Can you work these out from the model? Positions are in its coordinate system, mm. A direction names the side the tool comes from. Round coordinates to 2 decimals unless told otherwise and drop trailing zeros. Write each loop counter-clockwise with the first axis right and the second up, starting at its lowest first coordinate (ties: lowest second). Pieces come first, ordered by that corner, then holes. Notation, with made-up numbers: M 68,-22 L 123,-22 A14 ccw 123,-9 Z; hole C 52,48 d8. An arc over 180 degrees is marked long. Answer as a JSON object with one key per item and string values. Group by question number.
1) I'm going to push flat-ended pins straight in: pin 1 Ø6 at (x, z) = (-2, 7.5) entering from +Y; pin 2 Ø1 at (x, z) = (-2, 8.5) entering from -Y; pin 3 Ø5.5 at (x, y) = (-2, 4.5) entering from +Z; pin 4 Ø2 at (x, z) = (-6.5, 9.5) entering from -Y. Where does each tip first touch, or does it pass through?
2) Suppose I cut it at B-B, the plane y = -7.75. Write out the boundary of the cut face in (x, z).
3) Suppose I cut it at D-D, the plane z = 7. Write out the boundary of the cut face in (x, y), and give its area (3 significant figures).
4) Please list where these lines run through material, in increasing order: L1, parallel to Z at x = -6, y = -3.5; L2, parallel to X at y = -0.25, z = 21.5; L3, parallel to X at y = -5, z = 2 (3 decimals). Write a range as [from, to].
5) Suppose I cut it at C-C, the plane x = -6.25. Write out the boundary of the cut face in (y, z).
6) Suppose I cut it at A-A, the plane z = 2.5. Write out the boundary of the cut face in (x, y), and give its area (3 significant figures).
7) On a 3-axis mill with a long thin cutter (end or side, diameter ignored), from which of +Z, -Z, +X, -X, +Y, -Y can I reach the whole of each face in a straight line? I mean faces 1 (the flat face through (-8.665, -0.488, 1.972)), 2 (the cylindrical face through (-0.867, -3.905, 13.381)). Say none if no direction works.
from build123d import *

# Parameters (mm, degrees)
EXTRUDE_3_DEPTH = 4
SKETCH_3_R      = 4
EXTRUDE_4_DEPTH = 20
FILLET_1_R      = 1
FILLET_2_R      = 2


with BuildPart() as part:
    # 草图1 → 凸台-拉伸3 (new body)
    with BuildSketch(Plane.XY):
        Polygon((-8.337851922, -5.558416845), (0.644804231, -10), (8.982656153, -4.441583155), (8.337851922, 5.558416845), (-0.644804231, 10), (-8.982656153, 4.441583155), align=None)
    extrude(amount=EXTRUDE_3_DEPTH)

    # 草图3 → 凸台-拉伸4 (add)
    with BuildSketch(Plane.XY.offset(4)):
        Circle(SKETCH_3_R)
    extrude(amount=EXTRUDE_4_DEPTH)

    # 圆角1
    fillet_1_edges = [part.edges().sort_by_distance(p)[0] for p in [
        (-4, 0, 4),
    ]]
    fillet(fillet_1_edges, radius=FILLET_1_R)

    # 圆角2
    fillet_2_edges = [part.edges().sort_by_distance(p)[0] for p in [
        (-4, 0, 24),
    ]]
    fillet(fillet_2_edges, radius=FILLET_2_R)


solid = part.part
Results:
{
 "1": {"pin 1": "y = 4", "pin 2": "y = -3.71", "pin 3": "z = 23.99", "pin 4": "through"},
 "2": {"outline": "M -3.91,0 L 4.02,0 L 4.02,4 L -3.91,4 Z"},
 "3": {"outline": "C 0,0 d8", "area": "50.3 mm^2"},
 "4": {"L1": "[0, 4]", "L2": "[-3.99, 3.99]", "L3": "[-8.374, 8.145]"},
 "5": {"outline": "M -6.59,0 L 6.26,0 L 6.26,4 L -6.59,4 Z"},
 "6": {"outline": "M -8.98,4.44 L -8.34,-5.56 L 0.64,-10 L 8.98,-4.44 L 8.34,5.56 L -0.64,10 Z", "area": "261 mm^2"},
 "7": {"face 1": "+Z, -Z, -X, -Y", "face 2": "+Z"}
}
